Input: dimensioned drawing with shaded views. Units: mm. Origin: part minimum x, y, z. Give positions to 0.01 mm unless a question says otherwise; leave off trailing zeros. Write each loop counter-clockwise with the first axis right and the second up, starting at its lowest first coordinate (ties: lowest second). Pieces come first, ordered by that corner, then holes.
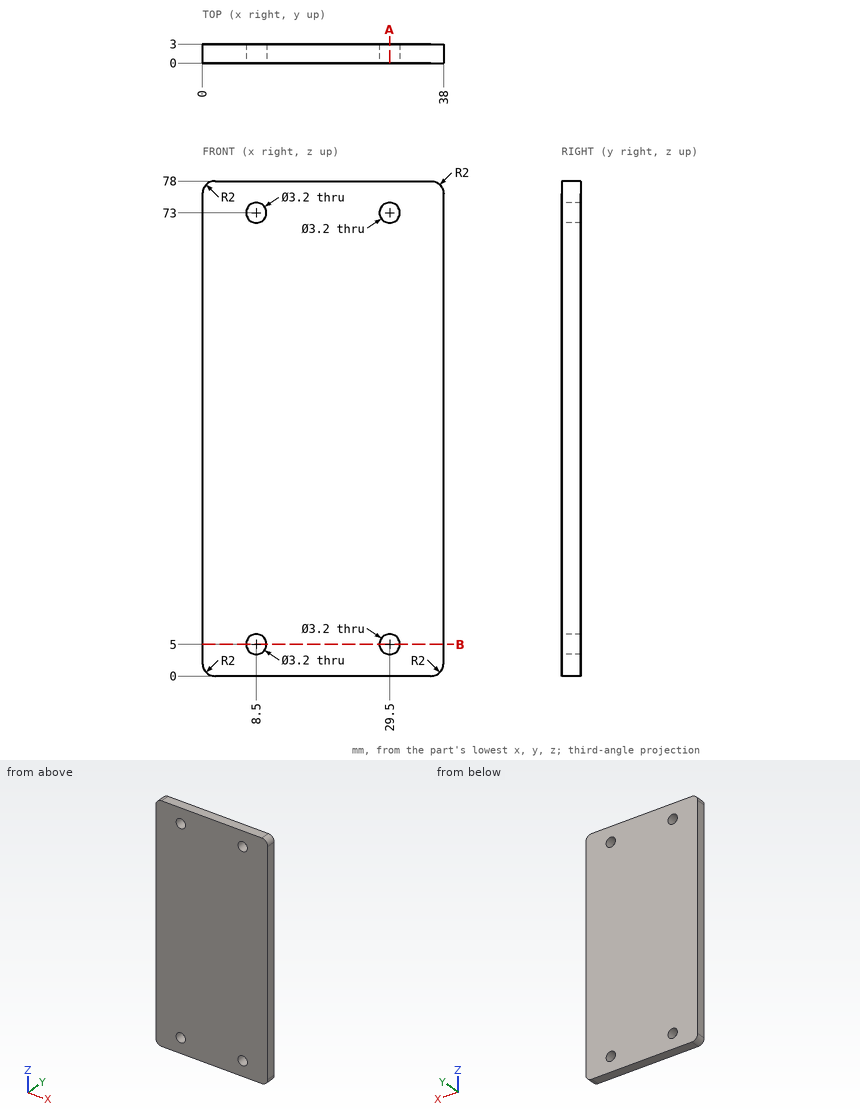
Item 1: Ray query, line 1 (Z direction, x = 8.5, y = 2.3); line 2 (X direction, y = 1.9, z = 5); line 3 (Z direction, x = 8, y = 1.3). Return the intervals inside material, ascending.
Item 2: Section A-A (x = 29.5). Return loops of the section in (y, z), and give its area (3 significant figures).
Item 3: Section B-B (z = 5). Return loops of the section in (x, y), and give its area (3 significant figures).
Solved:
1. line 1: z = 0 to 3.4, 6.6 to 71.4, 74.6 to 78
1. line 2: x = 0 to 6.9, 10.1 to 27.9, 31.1 to 38
1. line 3: z = 0 to 3.48, 6.52 to 71.48, 74.52 to 78
2. outline: (0, 0) - (3, 0) - (3, 3.4) - (0, 3.4) - close; (0, 6.6) - (3, 6.6) - (3, 71.4) - (0, 71.4) - close; (0, 74.6) - (3, 74.6) - (3, 78) - (0, 78) - close
2. area: 215 mm2
3. outline: (0, 0) - (6.9, 0) - (6.9, 3) - (0, 3) - close; (10.1, 0) - (27.9, 0) - (27.9, 3) - (10.1, 3) - close; (31.1, 0) - (38, 0) - (38, 3) - (31.1, 3) - close
3. area: 94.8 mm2
